```python
from build123d import *

# Parameters (mm, degrees)
SKETCH1_W           = 16
SKETCH1_H           = 12
BOSS_EXTRUDE1_DEPTH = 3
BOSS_EXTRUDE2_DEPTH = 11
CIRPATTERN2_COUNT   = 2
CIRPATTERN2_ANGLE   = 90


with BuildPart() as part:
    # Sketch1 → Boss-Extrude1 (new body)
    with BuildSketch(Plane.XY):
        with BuildLine():
            ThreePointArc((-4.875, 0), (-3.447145558, 3.447145558), (0, 4.875))
            Line((0, 4.875), (0, 6))
            Line((0, 6), (-8, 6))
            Line((-8, 6), (-8, 0))
            Line((-8, 0), (-4.875, 0))
        make_face()
        with BuildLine():
            ThreePointArc((0, -4.875), (-3.447145558, -3.447145558), (-4.875, 0))
            Line((-4.875, 0), (-8, 0))
            Line((-8, 0), (-8, -6))
            Line((-8, -6), (0, -6))
            Line((0, -6), (0, -4.875))
        make_face()
        with BuildLine():
            Line((0, -4.875), (0, 0))
            Line((0, 0), (-4.875, 0))
            ThreePointArc((-4.875, 0), (-3.447145558, -3.447145558), (0, -4.875))
        make_face()
        with BuildLine():
            Line((-4.875, 0), (0, 0))
            Line((0, 0), (0, 4.875))
            ThreePointArc((0, 4.875), (-3.447145558, 3.447145558), (-4.875, 0))
        make_face()
        with BuildLine():
            Line((0, 4.875), (0, 0))
            Line((0, 0), (0, -4.875))
            ThreePointArc((0, -4.875), (3.447145558, -3.447145558), (4.875, 0))
            ThreePointArc((4.875, 0), (3.447145558, 3.447145558), (0, 4.875))
        make_face()
        with BuildLine():
            Line((0, 6), (0, 4.875))
            ThreePointArc((0, 4.875), (3.447145558, 3.447145558), (4.875, 0))
            ThreePointArc((4.875, 0), (3.447145558, -3.447145558), (0, -4.875))
            Line((0, -4.875), (0, -6))
            Line((0, -6), (8, -6))
            Line((8, -6), (8, 6))
            Line((8, 6), (0, 6))
        make_face()
        with Locations((-16, 0)):
            Rectangle(SKETCH1_W, SKETCH1_H)
        with Locations((16, 0)):
            Rectangle(SKETCH1_W, SKETCH1_H)
    boss_extrude1 = extrude(amount=-BOSS_EXTRUDE1_DEPTH)

    # Sketch1_3 → Boss-Extrude2 (add)
    with BuildSketch(Plane.XY):
        with BuildLine():
            Line((-4.875, 0), (0, 0))
            Line((0, 0), (0, 4.875))
            ThreePointArc((0, 4.875), (-3.447145558, 3.447145558), (-4.875, 0))
        make_face()
        with BuildLine():
            Line((0, 4.875), (0, 0))
            Line((0, 0), (0, -4.875))
            ThreePointArc((0, -4.875), (3.447145558, -3.447145558), (4.875, 0))
            ThreePointArc((4.875, 0), (3.447145558, 3.447145558), (0, 4.875))
        make_face()
        with BuildLine():
            Line((0, -4.875), (0, 0))
            Line((0, 0), (-4.875, 0))
            ThreePointArc((-4.875, 0), (-3.447145558, -3.447145558), (0, -4.875))
        make_face()
    boss_extrude2 = extrude(amount=BOSS_EXTRUDE2_DEPTH)

    # CirPattern2: Boss-Extrude1, Boss-Extrude2 ×2 about axis
    cirpattern2_axis = Axis((0, 0, 17.25), (0, -1, 0))
    add([boss_extrude1.rotate(cirpattern2_axis, i * CIRPATTERN2_ANGLE / (CIRPATTERN2_COUNT - 1)) for i in range(1, CIRPATTERN2_COUNT)])
    add([boss_extrude2.rotate(cirpattern2_axis, i * CIRPATTERN2_ANGLE / (CIRPATTERN2_COUNT - 1)) for i in range(1, CIRPATTERN2_COUNT)])


solid = part.part
```
Model file for the job. Use its own axes, mm. A direction names the side the tool comes from. Give positions to 0.01 mm unless a question says otherwise; leave off trailing zeros. Write each loop counter-clockwise with the first axis right and the second up, starting at its lowest first coordinate (ties: lowest second). Pieces come first, ordered by that corner, then holes. Notation, with made-up numbers: (75, 35.5) - (96, 35.5) arc R15 cw to (96, 59.5) - close; hole circle Ø6 at (38, 16). An arc over 180 degrees is marked (long way). One line per question, with ' | ' between items. Start each with the question number.
(1) Slice it at B-B on x = 10.5. Write the cut outline in (y, z) (3 decimals).
(2) 3-axis set-ups, long thin cutter, end or side, ignore diameter. For faces 1 (the face through (-4, 0, -3)), 2 (the face through (20.25, 0, -5)), 3 (the face through (0, 0, 11)): which of +Z, -Z, +X, -X, +Y, -Y reach the whole face in a straight line?
(3) Wall check: line 1 along X through (y, z) = (0.25, 4); line 2 along Z through (x, y) = (-19, -3); line 3 along X through (y, z) = (5.75, 31). Give the ranges that are in metal, low to high. Write a range as from..to.
(4) Slice it at D-D on z = 19.5. Write the cut outline in (x, y), plus the area to 3 significant figures.
(5) Two-plate mould, pull along X, no slides. Class faces 4 (the face through (17.25, 4.1, 20.3)), 5 (the face through (17.25, 0, -5)), 6 (the face through (22, 0, -3)): +X half, -X half, draft (parallel to the pull), parting line (faces both ways), or undercut.
(6) Pin check, flat tips, straight feed: P1, Ø1, axis at x = -6.5, y = -4, coming from the +Z side; P2, Ø1, axis at y = -3, z = 34.5, coming from the -X side; P3, Ø4, axis at x = 6, y = 1.5, coming from the -Z side. Stop position of each tip, or through.
(7) Slice it at C-C on y = -2.5. Write the cut outline in (x, z), plus the area to 3 significant figures.
(8) Slice it at A-A on z = 6. Write the cut outline in (x, y) (3 decimals), plus the area to 3 significant figures.
Results below:
1) outline: (-6, -3) - (6, -3) - (6, 0) - (-6, 0) - close; circle Ø9.75 at (0, 17.25)
2) face 1: -Z, -X, +Y, -Y | face 2: -Z, +X, +Y, -Y | face 3: +Z, -X, +Y, -Y
3) line 1: -4.87..4.87, 17.25..20.25 | line 2: -3..0 | line 3: 17.25..20.25
4) outline: (6.25, -4.32) - (17.25, -4.32) - (17.25, -6) - (20.25, -6) - (20.25, 6) - (17.25, 6) - (17.25, 4.32) - (6.25, 4.32) - close | area: 131 mm^2
5) face 4: undercut | face 5: -X half | face 6: draft
6) P1: z = 0 | P2: x = 17.25 | P3: z = -3
7) outline: (-24, -3) - (17.25, -3) - (17.25, -6.75) - (20.25, -6.75) - (20.25, -3) - (24, -3) - (24, 0) - (20.25, 0) - (20.25, 41.25) - (17.25, 41.25) - (17.25, 21.44) - (6.25, 21.44) - (6.25, 13.06) - (17.25, 13.06) - (17.25, 0) - (4.19, 0) - (4.19, 11) - (-4.19, 11) - (-4.19, 0) - (-24, 0) - close | area: 463 mm^2
8) outline: circle Ø9.75 at (0, 0); (17.25, -6) - (20.25, -6) - (20.25, 6) - (17.25, 6) - close | area: 111 mm^2
